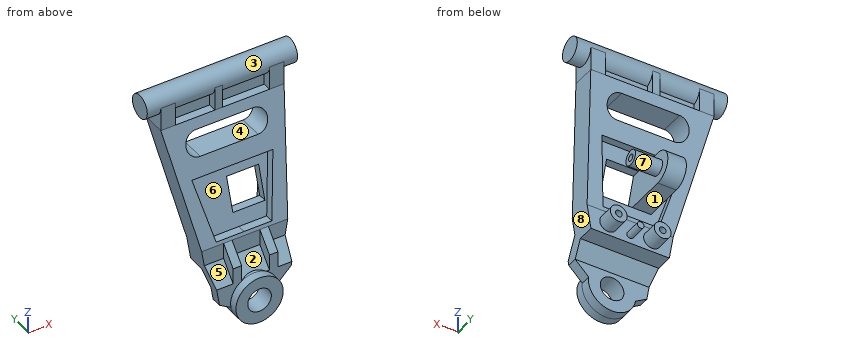
```python
from build123d import *

# Parameters (mm, degrees)
BOSS_EXTRUDE1_DEPTH             = 36.5
CUT_EXTRUDE1_DEPTH              = 76.543034093
CUT_EXTRUDE1_DEPTH_BACK         = 36.5
SKETCH2_R                       = 3.5
SKETCH2_W                       = 9.5
SKETCH2_H                       = 9.5
SKETCH5_W                       = 11.7
SKETCH5_H                       = 7
SKETCH5_W_2                     = 14
CUT_EXTRUDE2_DEPTH              = 2.5
SKETCH6_W                       = 14
SKETCH6_H                       = 7
SKETCH6_W_2                     = 11.7
CUT_EXTRUDE3_DEPTH              = 2.5
BOSS_EXTRUDE2_DEPTH             = 4
BOSS_EXTRUDE2_DEPTH_BACK        = 40.5
SKETCH3_R                       = 3.5
CUT_EXTRUDE4_REACH              = 79.555
CUT_EXTRUDE5_REACH              = 80.463
BOSS_EXTRUDE3_DEPTH             = 5.5
SKETCH10_R                      = 2.25
SKETCH10_R_2                    = 1
BOSS_EXTRUDE4_DEPTH             = 8
SKETCH11_R                      = 2.5
SKETCH11_R_2                    = 1
BOSS_EXTRUDE5_DEPTH             = 5
CUT_EXTRUDE7_DEPTH              = 12
CUT_EXTRUDE8_START              = 14.5
CUT_EXTRUDE8_DEPTH              = 8.25
CUT_EXTRUDE9_START              = 25.25
CUT_EXTRUDE9_DEPTH              = 8
SKETCH14_R                      = 7
SKETCH14_R_2                    = 3.5
BOSS_EXTRUDE6_DEPTH             = 2.5
BOSS_EXTRUDE6_DIRECTION_2_REACH = 82.238


with BuildPart() as part:
    # Sketch1 → Boss-Extrude1 (new body)
    with BuildSketch(Plane(origin=(0, 0, 0), x_dir=(0, 0, -1), z_dir=(1, 0, 0))):
        with BuildLine():
            Line((7, -3.5), (40.607142857, -14))
            Line((40.607142857, -14), (45.75, -18.5))
            Line((45.75, -18.5), (49.75, -18.5))
            Line((49.75, -18.5), (63.5, -18.5))
            Line((63.5, -18.5), (63.5, -15.5))
            Line((63.5, -15.5), (51.607142857, -15.5))
            Line((51.607142857, -15.5), (47.607142857, -12))
            Line((47.607142857, -12), (47.607142857, -7))
            Line((47.607142857, -7), (40.607142857, -7))
            Line((40.607142857, -7), (7, 3.5))
            Line((7, 3.5), (0, 3.5))
            ThreePointArc((0, 3.5), (-3.5, 0), (0, -3.5))
            Line((0, -3.5), (7, -3.5))
        make_face()
    extrude(amount=BOSS_EXTRUDE1_DEPTH)

    # Sketch2 → Cut-Extrude1 (cut, two sides: drawn at the far end of the back side and taken through both)
    with BuildSketch(Plane(origin=(0, 0, 0), x_dir=(1, 0, 0), z_dir=(0, 1, 0)).offset(-CUT_EXTRUDE1_DEPTH_BACK)):
        with Locations(Location((18.25, 56.5, 0), (0, 0, 90))):
            Circle(SKETCH2_R)
        with BuildLine():
            Line((25.192824074, 55.607142857), (29.192824074, 51.607142857))
            Line((29.192824074, 51.607142857), (36.5, 7))
            Line((36.5, 7), (46.5, 7))
            Line((46.5, 7), (46.5, 73.5))
            Line((46.5, 73.5), (-10, 73.5))
            Line((-10, 73.5), (-10, 7))
            Line((-10, 7), (0, 7))
            Line((0, 7), (7.962423087, 55.607142857))
            Line((7.962423087, 55.607142857), (11.338109181, 57.607142857))
            ThreePointArc((11.338109181, 57.607142857), (19.250119601, 63.428185966), (25.192824074, 55.607142857))
        make_face()
        with BuildLine():
            Line((9.678067434, 17), (26.821932566, 17))
            ThreePointArc((26.821932566, 17), (30.321932566, 13.5), (26.821932566, 10))
            Line((26.821932566, 10), (9.678067434, 10))
            ThreePointArc((9.678067434, 10), (6.178067434, 13.5), (9.678067434, 17))
        make_face()
        with Locations((22, 30.857142857)):
            Rectangle(SKETCH2_W, SKETCH2_H)
    extrude(amount=CUT_EXTRUDE1_DEPTH + CUT_EXTRUDE1_DEPTH_BACK, mode=Mode.SUBTRACT)

    # Sketch5 → Cut-Extrude2 (cut)
    with BuildSketch(Plane(origin=(0, 3.5, 0), x_dir=(1, 0, 0), z_dir=(0, 1, 0))):
        with Locations((10.15, 3.5)):
            Rectangle(SKETCH5_W, SKETCH5_H)
        with Locations((25.2, 3.5)):
            Rectangle(SKETCH5_W_2, SKETCH5_H)
    extrude(amount=-CUT_EXTRUDE2_DEPTH, mode=Mode.SUBTRACT)

    # Sketch6 → Cut-Extrude3 (cut)
    with BuildSketch(Plane.XZ.offset(3.5)):
        with Locations((25.2, -3.5)):
            Rectangle(SKETCH6_W, SKETCH6_H)
        with Locations((10.15, -3.5)):
            Rectangle(SKETCH6_W_2, SKETCH6_H)
    extrude(amount=-CUT_EXTRUDE3_DEPTH, mode=Mode.SUBTRACT)

    # Sketch3 → Boss-Extrude2 (add, two sides: drawn at the far end of the back side and taken through both)
    with BuildSketch(Plane(origin=(36.5, 0, 0), x_dir=(0, 0, -1), z_dir=(1, 0, 0)).offset(-BOSS_EXTRUDE2_DEPTH_BACK)):
        Circle(SKETCH3_R)
    extrude(amount=BOSS_EXTRUDE2_DEPTH + BOSS_EXTRUDE2_DEPTH_BACK)

    # Cut-Extrude4: up to this plane
    cut_extrude4_end = Plane(origin=(36.5, 0.954324111, -8.391680434), z_dir=(0, 0.9544980251192885, -0.2982172363284494))
    # Sketch7 → Cut-Extrude4 (cut, up to the surface)
    with BuildSketch(Plane(origin=(0, 0, 0), x_dir=(1, 0, 0), z_dir=(0, 1, 0)), mode=Mode.PRIVATE) as cut_extrude4_sk1:
        Polygon((18.222476089, 22.107142857), (30.222476089, 22.107142857), (26.498512221, 39.607142857), (18.248512221, 39.607142857), (9.998548743, 39.631691156), (6.222529213, 22.142849473), align=None)
    cut_extrude4_tool1 = split(extrude(cut_extrude4_sk1.sketch, amount=-CUT_EXTRUDE4_REACH, mode=Mode.PRIVATE), bisect_by=cut_extrude4_end, keep=Keep.BOTH, mode=Mode.PRIVATE)
    add(cut_extrude4_tool1.solids().sort_by_distance((18.234702, 0, -30.324637))[0], mode=Mode.SUBTRACT)

    # Cut-Extrude5: up to this plane
    cut_extrude5_end = Plane(origin=(36.5, -1.272837948, -7.695840216), z_dir=(0, 0.9544980251192885, -0.2982172363284494))
    # Sketch8 → Cut-Extrude5 (cut, up to the surface)
    with BuildSketch(Plane(origin=(0, -18.5, 0), x_dir=(1, 0, 0), z_dir=(0, 1, 0)), mode=Mode.PRIVATE) as cut_extrude5_sk1:
        Polygon((18.222476089, 22.107142857), (30.222476089, 22.107142857), (26.498512221, 39.607142857), (18.248512221, 39.607142857), (9.998548743, 39.631691156), (6.222529213, 22.142849473), align=None)
    cut_extrude5_tool1 = split(extrude(cut_extrude5_sk1.sketch, amount=CUT_EXTRUDE5_REACH, mode=Mode.PRIVATE), bisect_by=cut_extrude5_end, keep=Keep.BOTH, mode=Mode.PRIVATE)
    add(cut_extrude5_tool1.solids().sort_by_distance((18.234702, -18.5, -30.324637))[0], mode=Mode.SUBTRACT)

    # Sketch9 → Boss-Extrude3 (add)
    with BuildSketch(Plane(origin=(17.25, 0, 0), x_dir=(0, 0, -1), z_dir=(1, 0, 0))):
        with BuildLine():
            Line((26.107142857, -4.580581258), (26.107142857, 4.419418742))
            ThreePointArc((26.107142857, 4.419418742), (30.857142857, 9.169418742), (35.607142857, 4.419418742))
            Line((35.607142857, 4.419418742), (35.607142857, -7.548700281))
            Line((35.607142857, -7.548700281), (26.107142857, -4.580581258))
        make_face()
    extrude(amount=-BOSS_EXTRUDE3_DEPTH)

    # Sketch10 → Boss-Extrude4 (add)
    with BuildSketch(Plane(origin=(17.25, 0, 0), x_dir=(0, 0, -1), z_dir=(1, 0, 0))):
        with Locations((30.857142857, 4.419418742)):
            Circle(SKETCH10_R)
        with Locations((30.857142857, 4.419418742)):
            Circle(SKETCH10_R_2, mode=Mode.SUBTRACT)
    extrude(amount=BOSS_EXTRUDE4_DEPTH)

    # Sketch11 → Boss-Extrude5 (add)
    # profile 1 of 3: a face of its own
    with BuildSketch(Plane(origin=(0, -7, 0), x_dir=(1, 0, 0), z_dir=(0, 1, 0))):
        with Locations(Location((11.75, 44.107142857, 0), (0, 0, 90))):
            Circle(SKETCH11_R)
        with Locations(Location((11.75, 44.107142857, 0), (0, 0, 270))):
            Circle(SKETCH11_R_2, mode=Mode.SUBTRACT)
    # profile 2 of 3: a face of its own
    with BuildSketch(Plane(origin=(0, -7, 0), x_dir=(1, 0, 0), z_dir=(0, 1, 0))):
        with Locations(Location((18.25, 45.107142857, 0), (0, 0, 90))):
            Circle(SKETCH11_R_2)
    # profile 3 of 3: a face of its own
    with BuildSketch(Plane(origin=(0, -7, 0), x_dir=(1, 0, 0), z_dir=(0, 1, 0))):
        with Locations(Location((24.75, 44.107142857, 0), (0, 0, 90))):
            Circle(SKETCH11_R)
        with Locations(Location((24.75, 44.107142857, 0), (0, 0, 90))):
            Circle(SKETCH11_R_2, mode=Mode.SUBTRACT)
    extrude(amount=BOSS_EXTRUDE5_DEPTH)

    # Sketch13 → Cut-Extrude7 (cut)
    with BuildSketch(Plane(origin=(0, 0, 0), x_dir=(0, 0, -1), z_dir=(1, 0, 0))):
        Polygon((53.908508937, -21.5), (45.337080366, -14), (40.607142857, -14), (40.607142857, -21.5), align=None)
    extrude(amount=CUT_EXTRUDE7_DEPTH, mode=Mode.SUBTRACT)

    # Sketch13<3> → Cut-Extrude8 (cut)
    with BuildSketch(Plane(origin=(0, 0, 0), x_dir=(0, 0, -1), z_dir=(1, 0, 0)).offset(CUT_EXTRUDE8_START)):
        Polygon((53.908508937, -21.5), (45.337080366, -14), (40.607142857, -14), (40.607142857, -21.5), align=None)
    extrude(amount=CUT_EXTRUDE8_DEPTH, mode=Mode.SUBTRACT)

    # Sketch13<4> → Cut-Extrude9 (cut)
    with BuildSketch(Plane(origin=(0, 0, 0), x_dir=(0, 0, -1), z_dir=(1, 0, 0)).offset(CUT_EXTRUDE9_START)):
        Polygon((53.908508937, -21.5), (45.337080366, -14), (40.607142857, -14), (40.607142857, -21.5), align=None)
    extrude(amount=CUT_EXTRUDE9_DEPTH, mode=Mode.SUBTRACT)

    # Sketch14 → Boss-Extrude6 (add)
    with BuildSketch(Plane.XZ.offset(18.5)):
        with Locations(Location((18.25, -56.5, 0), (0, 0, 270))):
            Circle(SKETCH14_R)
        with Locations(Location((18.25, -56.5, 0), (0, 0, 270))):
            Circle(SKETCH14_R_2, mode=Mode.SUBTRACT)
    extrude(amount=BOSS_EXTRUDE6_DEPTH)

    # Boss-Extrude6 direction 2: up to this face of the body (flat: up to its plane)
    boss_extrude6_direction_2_end = Plane(part.part.faces().sort_by_distance((27.530853261, -16.180546647, -47.829133677))[0])
    # Sketch14 → Boss-Extrude6 direction 2 (add, up to the picked face)
    with BuildSketch(Plane.XZ.offset(18.5), mode=Mode.PRIVATE) as boss_extrude6_direction_2_sk1:
        with Locations(Location((18.25, -56.5, 0), (0, 0, 270))):
            Circle(SKETCH14_R)
        with Locations(Location((18.25, -56.5, 0), (0, 0, 270))):
            Circle(SKETCH14_R_2, mode=Mode.SUBTRACT)
    boss_extrude6_direction_2_tool1 = split(extrude(boss_extrude6_direction_2_sk1.sketch, amount=-BOSS_EXTRUDE6_DIRECTION_2_REACH, mode=Mode.PRIVATE), bisect_by=boss_extrude6_direction_2_end, keep=Keep.BOTH, mode=Mode.PRIVATE)
    add(boss_extrude6_direction_2_tool1.solids().sort_by(Axis((18.25, -18.5, -49.69799), (0, 1, 0)))[0])


solid = part.part
```
Here's how the part is built. I have some questions about the finished solid (model axes, mm). Face numbers are marked on the shaded views. A direction names the side the tool comes from. Give positions to 0.01 mm unless a question says otherwise; leave off trailing zeros. Loops run counter-clockwise (first coordinate to the right, second up) from the corner with the lowest first, then second, coordinate; pieces in that order, holes last. Notation, with made-up numbers: (46.5, -27) -> (71.5, -27) arc R7 cw to (71.5, -15) -> close; hole circle Ø11 at (-25, 46). An arc over 180 degrees is marked (long way). Use one line per item in the form item = value. Start each with the question number.
1) Imagine slicing it at D-D (z = -2). Please give me the cut outline in (x, y), then the cut area to 3 significant figures.
2) Which directions (+Z, -Z, +X, -X, +Y, -Y) give clear straight access to the entire face, cutting with the end or side of a thin tool? Please do the marked faces 1, 2, 3, 4 and 5.
3) Please list where these lines run through material, in increasing order: line 1 along X through (y, z) = (-18.1, -56.5); line 2 along X through (y, z) = (-1, -11); line 3 along Z through (x, y) = (22.5, -3).
4) Imagine slicing it at A-A (z = -27). Please give me the cut outline in (x, y).
5) Imagine slicing it at B-B (x = -1). Please give me the cut outline in (y, z).
6) Thinking about a two-plate mould opening in X: for the marked faces 6, 7 and 8, which applies, +X half, -X half, draft (parallel to the pull), parting line (faces both ways), or undercut?
7) For P1, Ø1.7, axis at x = 23, y = -2, coming from the -Z side; P2, Ø4.5, axis at x = 35, z = -5, coming from the +Y side; P3, Ø3, axis at y = 1.5, z = -29, coming from the -X side; P4, Ø0.8, axis at y = -2, z = -3, coming from the +X side, each with a flat end and sliding along its axis, tell me the tip position at first contact or that it passes through.
8) Imagine slicing it at C-C (z = -13.5). Please give me the cut outline in (x, y), then the cut area to 3 significant figures.
Check values:
q1.outline = (-4, -2.87) -> (0, -2.87) -> (0, -3.5) -> (4.3, -3.5) -> (4.3, -2.87) -> (16, -2.87) -> (16, -3.5) -> (18.2, -3.5) -> (18.2, -2.87) -> (32.2, -2.87) -> (32.2, -3.5) -> (36.5, -3.5) -> (36.5, -2.87) -> (40.5, -2.87) -> (40.5, 2.87) -> (36.5, 2.87) -> (36.5, 3.5) -> (32.2, 3.5) -> (32.2, 2.87) -> (18.2, 2.87) -> (18.2, 3.5) -> (16, 3.5) -> (16, 2.87) -> (4.3, 2.87) -> (4.3, 3.5) -> (0, 3.5) -> (0, 2.87) -> (-4, 2.87) -> close
q1.area = 269 mm^2
q2.face_1 = +Y
q2.face_2 = +Z, -Y
q2.face_3 = none
q2.face_4 = +Y, -Y
q2.face_5 = +Z, -X, -Y
q3.line_1 = 9.47 to 14.75, 21.75 to 25.25
q3.line_2 = 0.66 to 7.23, 29.27 to 35.84
q3.line_3 = -45.2 to -43.02, -22.11 to -17, -10 to -7, -1.8 to 1.8
q4.outline = (3.28, -9.75) -> (7.27, -9.75) -> (7.27, -7.3) -> (17.25, -7.3) -> (17.25, 7.19) -> (11.75, 7.19) -> (11.75, -4.86) -> (7.27, -4.86) -> (7.27, -2.75) -> (3.28, -2.75) -> close; (26.75, -7.3) -> (29.18, -7.3) -> (29.18, -9.75) -> (33.22, -9.75) -> (33.22, -2.75) -> (29.18, -2.75) -> (29.18, -4.86) -> (26.75, -4.86) -> close
q5.outline = circle Ø7 at (0, 0)
q6.face_6 = undercut
q6.face_7 = draft
q6.face_8 = +X half
q7.P1 = -46.44
q7.P2 = 3.5
q7.P3 = 11.75
q7.P4 = 40.5
q8.outline = (1.06, -5.53) -> (6.18, -5.53) -> (6.18, 1.47) -> (1.06, 1.47) -> close; (30.32, -5.53) -> (35.44, -5.53) -> (35.44, 1.47) -> (30.32, 1.47) -> close
q8.area = 71.6 mm^2
